For this review, take the finished solid that the model builds, in its own axes (mm). A direction names the side the tool comes from. Give positions to 0.01 mm unless a question says otherwise; leave off trailing zeros. Order: outer loops, then holes, each group sorted by start corner. A loop starts at its lowest first (then second) coordinate and runs counter-clockwise, first axis right, second up.
Item 1: For probe 1 along X at (y, z) = (52.5, 1.2) (1 decimal); probe 2 along X at (y, z) = (17, 1.4) (3 decimals); probe 3 along X at (y, z) = (4, 2.3) (3 decimals), list the stretches that pass through material, from the lowest coordinate up.
Item 2: For P1, Ø5, axis at x = -36.5, y = 37, coming from the -Z side; P2, Ø1.6, axis at y = 62.5, z = 2, coming from the +X side, all flat-tipped, find the tip position at first contact; note any pin that passes through.
Item 3: Machinability: for faces 5 (the flat face through (-57, -15.875, 2)), 6 (the flat face through (60.325, -37, 2)), 7 (the flat face through (62, 30.162, 2)), 8 (the flat face through (30.162, -62, 2)), 9 (the flat face through (45, 51.594, 2)), which of the approach directions +Z, -Z, +X, -X, +Y, -Y give a long, thin tool a straight path to every point of the face, cutting with its end or side? Answer none if there is none.
Item 4: The part is to be moulded in two halves that separate along Y. For faces 1 (the flat face through (-23, 60.325, 2)), 2 (the flat face through (30.162, 62, 2)), 3 (the flat face through (-62, 0, 2)), 4 (the flat face through (45, -63.5, 2)), say which applies: released by +Y, released by -Y, zero draft, split by the parting line, or undercut.
Item 5: Consider section C-C (z = 2.25). Give the number of separate pieces and of enclosed holes in the cut face, plus the area to 3 significant figures.
Item 6: Consider section A-A (x = 35.5). Give the boundary of the cut face in (y, z) (3 decimals), plus the area to 3 significant figures.
```python
from build123d import *

# Parameters (mm, degrees)
BOSS_EXTRUDE1_DEPTH = 3.175
SKETCH2_R           = 0.79375
CUT_EXTRUDE1_DEPTH  = 90.858670283


with BuildPart() as part:
    # Sketch1 → Boss-Extrude1 (new body)
    with BuildSketch(Plane.XY):
        Polygon((-60.325, 60.325), (-60.325, 63.5), (-30.1625, 63.5), (-30.1625, 60.325), (0, 60.325), (0, 63.5), (30.1625, 63.5), (30.1625, 60.325), (60.325, 60.325), (63.5, 60.325), (63.5, 30.1625), (60.325, 30.1625), (60.325, 0), (63.5, 0), (63.5, -30.1625), (60.325, -30.1625), (60.325, -60.325), (60.325, -63.5), (30.1625, -63.5), (30.1625, -60.325), (0, -60.325), (0, -63.5), (-30.1625, -63.5), (-30.1625, -60.325), (-60.325, -60.325), (-63.5, -60.325), (-63.5, -30.1625), (-60.325, -30.1625), (-60.325, 0), (-63.5, 0), (-63.5, 30.1625), (-60.325, 30.1625), align=None)
    extrude(amount=BOSS_EXTRUDE1_DEPTH)

    # Sketch2 → Cut-Extrude1 (cut, through all)
    with BuildSketch(Plane.XY.offset(3.175)):
        Polygon((-14.2875, 53.975), (-14.2875, 60.325), (-15.875, 60.325), (-15.875, 53.975), (-17.4625, 53.975), (-17.4625, 51.59375), (-12.7, 51.59375), (-12.7, 53.975), align=None)
        Polygon((-53.975, 46.0375), (-60.325, 46.0375), (-60.325, 44.45), (-53.975, 44.45), (-53.975, 42.8625), (-51.59375, 42.8625), (-51.59375, 47.625), (-53.975, 47.625), align=None)
        Polygon((46.0375, 60.325), (44.45, 60.325), (44.45, 53.975), (42.8625, 53.975), (42.8625, 51.59375), (47.625, 51.59375), (47.625, 53.975), (46.0375, 53.975), align=None)
        Polygon((60.325, 14.2875), (60.325, 15.875), (53.975, 15.875), (53.975, 17.4625), (51.59375, 17.4625), (51.59375, 12.7), (53.975, 12.7), (53.975, 14.2875), align=None)
        Polygon((-53.975, -14.2875), (-60.325, -14.2875), (-60.325, -15.875), (-53.975, -15.875), (-53.975, -17.4625), (-51.59375, -17.4625), (-51.59375, -12.7), (-53.975, -12.7), align=None)
        Polygon((-46.0375, -53.975), (-46.0375, -60.325), (-44.45, -60.325), (-44.45, -53.975), (-42.8625, -53.975), (-42.8625, -51.59375), (-47.625, -51.59375), (-47.625, -53.975), align=None)
        Polygon((60.325, -46.0375), (60.325, -44.45), (53.975, -44.45), (53.975, -42.8625), (51.59375, -42.8625), (51.59375, -47.625), (53.975, -47.625), (53.975, -46.0375), align=None)
        Polygon((14.2875, -60.325), (15.875, -60.325), (15.875, -53.975), (17.4625, -53.975), (17.4625, -51.59375), (12.7, -51.59375), (12.7, -53.975), (14.2875, -53.975), align=None)
        with Locations((-45.24375, 61.9125)):
            Circle(SKETCH2_R)
        with Locations((15.08125, 61.9125)):
            Circle(SKETCH2_R)
        with Locations((61.9125, 45.24375)):
            Circle(SKETCH2_R)
        with Locations((61.9125, -15.08125)):
            Circle(SKETCH2_R)
        with Locations((45.24375, -61.9125)):
            Circle(SKETCH2_R)
        with Locations((-15.08125, -61.9125)):
            Circle(SKETCH2_R)
        with Locations((-61.9125, -45.24375)):
            Circle(SKETCH2_R)
        with Locations((-61.9125, 15.08125)):
            Circle(SKETCH2_R)
    extrude(amount=-CUT_EXTRUDE1_DEPTH, mode=Mode.SUBTRACT)


solid = part.part
```
Resolved:
1. probe 1: x = -60.3 to -17.5, -12.7 to 42.9, 47.6 to 63.5
1. probe 2: x = -63.5 to 51.594, 53.975 to 60.325
1. probe 3: x = -63.5 to 60.325
2. P1: stops at z = 0
2. P2: stops at x = 30.16
3. face 5: +Z, -Z, -X
3. face 6: +Z, -Z, +X, -Y
3. face 7: +Z, -Z, +X
3. face 8: +Z, -Z, -Y
3. face 9: +Z, -Z
4. face 1: released by +Y
4. face 2: zero draft
4. face 3: undercut
4. face 4: released by -Y
5. separate pieces: 1
5. enclosed holes: 8
5. area: 15,100 mm2
6. outline: (-63.5, 0) - (60.325, 0) - (60.325, 3.175) - (-63.5, 3.175) - close
6. area: 393 mm2
